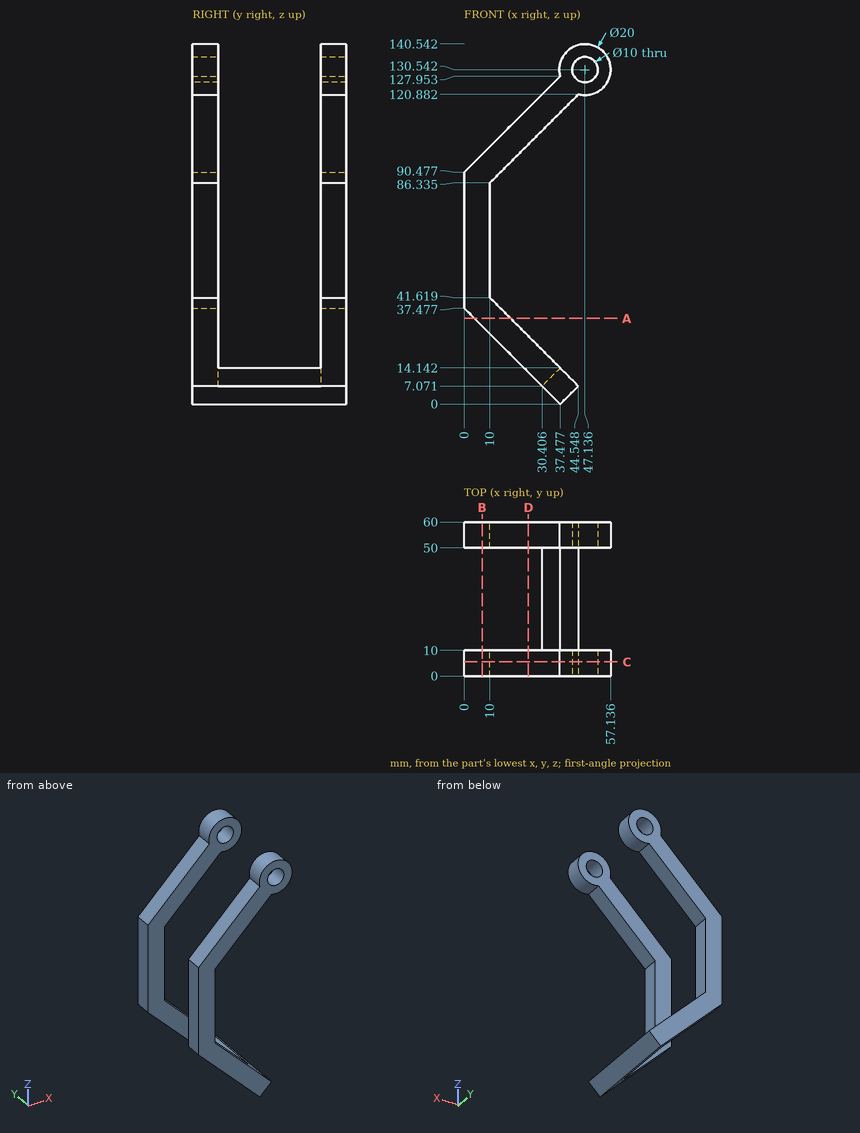
Input: dimensioned drawing with shaded views. Units: mm. Origin: part minimum x, y, z. Give positions to 0.01 mm unless a question says otherwise; leave off trailing zeros. Loops run counter-clockwise (first coordinate to the right, second up) from the corner with the lowest first, then second, coordinate; pieces in that order, holes last. Notation, with made-up numbers: M -3.5,26 L 13.5,26 A12 ccw 13.5,32 Z; hole C 5,-13.75 d4. An arc over 180 degrees is marked long. Put each result on its own line as item: value.
1) Material intervals for L1, parallel to X at y = 9, z = 61; L2, parallel to Z at x = 37, y = 9.5 (1 decimal); L3, parallel to Z at x = 35, y = 11 (1 decimal), sorted ascending. Write a range as from..to.
Computed values:
L1: x = 0..10
L2: z = 0.5..14.6, 113.3..127.5
L3: z = 2.5..11.7
2) Cut plane B-B, the plane x = 7. Return the cut outline in (y, z).
Computed values:
outline: M 0,30.48 L 10,30.48 L 10,97.48 L 0,97.48 Z; M 50,30.48 L 60,30.48 L 60,97.48 L 50,97.48 Z
3) First-contact query: P1, Ø6, axis at x = 28, y = 45, coming from the -Z side (1 decimal); P2, Ø8, axis at x = 23, y = 45.5, coming from the +Z side; P3, Ø6, axis at y = 50.5, z = 15.5, coming from the +X side; P4, Ø3, axis at y = 56.5, z = 72.5, coming from the +X side. Flat tips, straight axial feed; report the tip coordinate or a pass-through.
Computed values:
P1: stops at z = 6.5
P2: passes through
P3: stops at x = 39.12
P4: stops at x = 10
4) Cut plane C-C, the plane y = 5.5. Return the cut outline in (x, z) (1 decimal).
Computed values:
outline: M 0,37.5 L 37.5,0 L 44.5,7.1 L 10,41.6 L 10,86.3 L 44.5,120.9 A10 ccw long 37.5,128 L 0,90.5 Z; hole C 47.1,130.5 d10
5) Cut plane D-D, the plane x = 25. Return the cut outline in (y, z) (1 decimal).
Computed values:
outline: M 0,12.5 L 10,12.5 L 10,26.6 L 0,26.6 Z; M 0,101.3 L 10,101.3 L 10,115.5 L 0,115.5 Z; M 50,12.5 L 60,12.5 L 60,26.6 L 50,26.6 Z; M 50,101.3 L 60,101.3 L 60,115.5 L 50,115.5 Z
6) Cut plane A-A, the plane z = 33.5. Return the cut outline in (x, y), plus the area to 3 significant figures.
Computed values:
outline: M 3.98,0 L 18.12,0 L 18.12,10 L 3.98,10 Z; M 3.98,50 L 18.12,50 L 18.12,60 L 3.98,60 Z
area: 283 mm^2
